For this review, use the dimensioned drawing (mm, ordinates from the lowest corner) and the shaded views. A direction names the side the tool comes from. Coordinates: 2 decimals unless noted, no trailing zeros. Loops run counter-clockwise (first coordinate to the right, second up) from the corner with the lowest first, then second, coordinate; pieces in that order, holes last. Notation, with made-up numbers: (-39, 9.25) - (4, 9.25) arc R25 cw to (4, 34.25) - close; hole circle Ø11 at (44.25, -14.5). An arc over 180 degrees is marked (long way). Use one line per item in the form item = value. Start each with the question number.
(1) Tool access review of the marked faces 1 and 2: name each direction out of +Z, -Z, +X, -X, +Y, -Y from which nothing blocks a thin tool from reaching the whole face with its end or side.
(2) Add section C-C (x = 15). State the section outline as (y, z) points.
(3) For L1, parallel to Z at x = 1, y = 14; L2, parallel to Y at x = 15, z = 24.5; L3, parallel to X at y = 14, z = 16, list the stretches that pass through material, from the lowest coordinate up.
(4) Add section B-B (y = 14). State the section outline as (x, z) points, plus the area to 3 significant figures.
(5) Add section D-D (z = 27.5). State the section outline as (x, y) points.
(6) Add section A-A (z = 20). State the section outline as (x, y) points, plus the area to 3 significant figures.
(7) The part is to be moulded in two halves that separate along X. For the marked faces 3, 4 and 5, say which applies: pulls with the +X half, pulls with the -X half, needs draft (parallel to the pull), parting line crosses it, or undercut.
(8) Clearance check with flat-ended pins moving along their axes: pin 1 Ø20 at (x, z) = (57.5, 16) entering from -Y; pin 2 Ø4.5 at (y, z) = (14, 8) entering from +X; pin 3 Ø8 at (x, z) = (50, 20) entering from -Y. State where each tip first meets the part, or that it passes through.
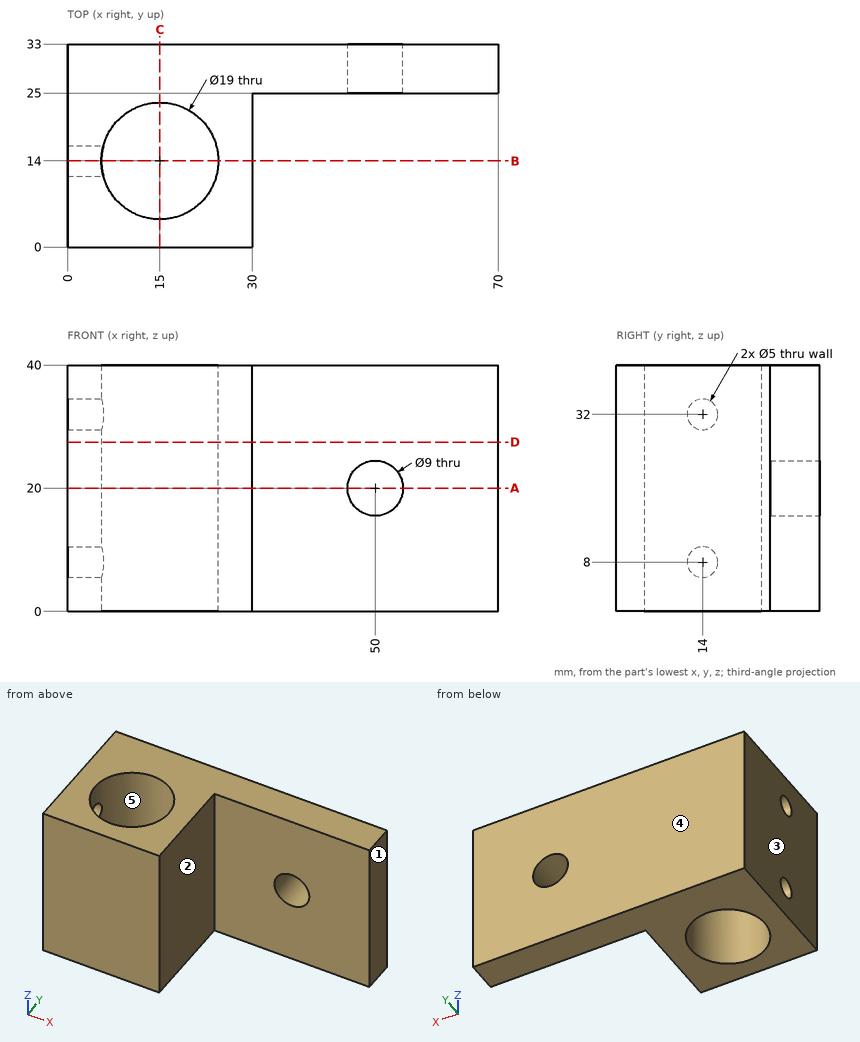
Computed values:
q1.face_1 = +Z, -Z, +X, +Y, -Y
q1.face_2 = +Z, -Z, +X, -Y
q2.outline = (0, 0) - (4.5, 0) - (4.5, 40) - (0, 40) - close; (23.5, 0) - (33, 0) - (33, 40) - (23.5, 40) - close
q3.L1 = 0 to 5.5, 10.5 to 29.5, 34.5 to 40
q3.L2 = 0 to 4.5, 23.5 to 33
q3.L3 = 0 to 5.5, 24.5 to 30
q4.outline = (0, 0) - (5.5, 0) - (5.5, 5.5) - (0, 5.5) - close; (0, 10.5) - (5.5, 10.5) - (5.5, 29.5) - (0, 29.5) - close; (0, 34.5) - (5.5, 34.5) - (5.5, 40) - (0, 40) - close; (24.5, 0) - (30, 0) - (30, 40) - (24.5, 40) - close
q4.area = 385 mm^2
q5.outline = (0, 0) - (30, 0) - (30, 25) - (70, 25) - (70, 33) - (0, 33) - close; hole circle Ø19 at (15, 14)
q6.outline = (0, 0) - (30, 0) - (30, 25) - (45.5, 25) - (45.5, 33) - (0, 33) - close; (54.5, 25) - (70, 25) - (70, 33) - (54.5, 33) - close; hole circle Ø19 at (15, 14)
q6.area = 954 mm^2
q7.face_3 = pulls with the -X half
q7.face_4 = needs draft
q7.face_5 = undercut
q8.pin_1 = 25
q8.pin_2 = 30
q8.pin_3 = through
